from build123d import *

# Parameters (mm, degrees)
BOSS_EXTRU_1_DEPTH      = 6
ESQUISSE3_R             = 19
ENL_V_MAT_EXTRU_1_DEPTH = 10
ESQUISSE4_W             = 20
ESQUISSE4_H             = 60
ENL_V_MAT_EXTRU_2_DEPTH = 10
ESQUISSE5_W             = 20
ESQUISSE5_H             = 48
BOSS_EXTRU_2_DEPTH      = 6
ESQUISSE6_R             = 1.5
ENL_V_MAT_EXTRU_3_DEPTH = 10
ESQUISSE7_R             = 1.5
ENL_V_MAT_EXTRU_4_DEPTH = 10
ESQUISSE8_R             = 1.5
ENL_V_MAT_EXTRU_5_DEPTH = 10
ESQUISSE9_R             = 3.5
ESQUISSE9_R_2           = 1.5
ENL_V_MAT_EXTRU_6_DEPTH = 10
ESQUISSE10_R            = 1.5
ENL_V_MAT_EXTRU_7_DEPTH = 10
ESQUISSE11_R            = 1.5
ENL_V_MAT_EXTRU_8_DEPTH = 10
ESQUISSE13_R            = 5
ENL_V_MAT_EXTRU_9_DEPTH = 10


with BuildPart() as part:
    # Esquisse2 → Boss.-Extru.1 (new body)
    with BuildSketch(Plane.XY):
        Polygon((-82.846139514, -43.409107348), (-62.846139514, -43.409107348), (-62.846139514, -37.409107348), (-42.846139514, -37.409107348), (-42.846139514, -43.409107348), (-22.846139514, -43.409107348), (-22.846139514, -37.409107348), (-2.846139514, -37.409107348), (-2.846139514, -43.409107348), (17.153860486, -43.409107348), (17.153860486, -37.409107348), (37.153860486, -37.409107348), (37.153860486, -43.409107348), (57.153860486, -43.409107348), (57.153860486, -37.409107348), (77.153860486, -37.409107348), (77.153860486, -43.409107348), (97.153860486, -43.409107348), (97.153860486, -37.409107348), (117.153860486, -37.409107348), (117.153860486, -43.409107348), (137.153860486, -43.409107348), (137.153860486, -37.409107348), (157.153860486, -37.409107348), (157.153860486, -43.409107348), (177.153860486, -43.409107348), (177.153860486, -37.409107348), (197.153860486, -37.409107348), (197.153860486, -43.409107348), (217.153860486, -43.409107348), (217.153860486, -37.409107348), (237.153860486, -37.409107348), (237.153860486, -43.409107348), (257.153860486, -43.409107348), (257.153860486, -37.409107348), (277.153860486, -37.409107348), (277.153860486, -43.409107348), (297.153860486, -43.409107348), (297.153860486, -37.409107348), (317.153860486, -37.409107348), (317.153860486, -43.409107348), (337.153860486, -43.409107348), (337.153860486, 16.590892652), (317.153860486, 16.590892652), (317.153860486, 10.590892652), (297.153860486, 10.590892652), (297.153860486, 16.590892652), (277.153860486, 16.590892652), (277.153860486, 10.590892652), (257.153860486, 10.590892652), (257.153860486, 16.590892652), (237.153860486, 16.590892652), (237.153860486, 10.590892652), (217.153860486, 10.590892652), (217.153860486, 16.590892652), (197.153860486, 16.590892652), (197.153860486, 10.590892652), (177.153860486, 10.590892652), (177.153860486, 16.590892652), (157.153860486, 16.590892652), (157.153860486, 10.590892652), (137.153860486, 10.590892652), (137.153860486, 16.590892652), (117.153860486, 16.590892652), (117.153860486, 10.590892652), (97.153860486, 10.590892652), (97.153860486, 16.590892652), (77.153860486, 16.590892652), (77.153860486, 10.590892652), (57.153860486, 10.590892652), (57.153860486, 16.590892652), (37.153860486, 16.590892652), (37.153860486, 10.590892652), (17.153860486, 10.590892652), (17.153860486, 16.590892652), (-2.846139514, 16.590892652), (-2.846139514, 10.590892652), (-22.846139514, 10.590892652), (-22.846139514, 16.590892652), (-42.846139514, 16.590892652), (-42.846139514, 10.590892652), (-62.846139514, 10.590892652), (-62.846139514, 16.590892652), (-82.846139514, 16.590892652), align=None)
    extrude(amount=BOSS_EXTRU_1_DEPTH)

    # Esquisse3 → Enlèv. mat.-Extru.1 (cut)
    with BuildSketch(Plane.XY.offset(6)):
        with Locations((-37.846139514, -13.409107348)):
            Circle(ESQUISSE3_R)
    extrude(amount=-ENL_V_MAT_EXTRU_1_DEPTH, mode=Mode.SUBTRACT)

    # Esquisse4 → Enlèv. mat.-Extru.2 (cut)
    with BuildSketch(Plane.XY.offset(6)):
        with Locations((-72.846139514, -13.409107348)):
            Rectangle(ESQUISSE4_W, ESQUISSE4_H)
    extrude(amount=-ENL_V_MAT_EXTRU_2_DEPTH, mode=Mode.SUBTRACT)

    # Esquisse5 → Boss.-Extru.2 (add)
    with BuildSketch(Plane.XY.offset(6)):
        with Locations((347.153860486, -13.409107348)):
            Rectangle(ESQUISSE5_W, ESQUISSE5_H)
    extrude(amount=-BOSS_EXTRU_2_DEPTH)

    # Esquisse6 → Enlèv. mat.-Extru.3 (cut)
    with BuildSketch(Plane.XY.offset(6)):
        with Locations((127.153860486, -40.409107348)):
            Circle(ESQUISSE6_R)
        with Locations((287.153860486, -40.409107348)):
            Circle(ESQUISSE6_R)
        with Locations((7.153860486, -40.409107348)):
            Circle(ESQUISSE6_R)
        with Locations((7.153860486, 13.590892652)):
            Circle(ESQUISSE6_R)
        with Locations((127.153860486, 13.590892652)):
            Circle(ESQUISSE6_R)
        with Locations((287.153860486, 13.590892652)):
            Circle(ESQUISSE6_R)
    extrude(amount=-ENL_V_MAT_EXTRU_3_DEPTH, mode=Mode.SUBTRACT)

    # Esquisse7 → Enlèv. mat.-Extru.4 (cut)
    with BuildSketch(Plane.XY.offset(6)):
        with Locations((-59.846139514, -13.409107348)):
            Circle(ESQUISSE7_R)
    extrude(amount=-ENL_V_MAT_EXTRU_4_DEPTH, mode=Mode.SUBTRACT)

    # Esquisse8 → Enlèv. mat.-Extru.5 (cut)
    with BuildSketch(Plane.XY.offset(6)):
        with Locations((354.153860486, -13.409107348)):
            Circle(ESQUISSE8_R)
    extrude(amount=-ENL_V_MAT_EXTRU_5_DEPTH, mode=Mode.SUBTRACT)

    # Esquisse9 → Enlèv. mat.-Extru.6 (cut)
    with BuildSketch(Plane.XY.offset(6)):
        with Locations((1.153860486, -13.409107348)):
            Circle(ESQUISSE9_R)
        with Locations((-7.096139514, -13.409107348)):
            Circle(ESQUISSE9_R_2)
        with Locations((9.403860486, -13.409107348)):
            Circle(ESQUISSE9_R_2)
    extrude(amount=-ENL_V_MAT_EXTRU_6_DEPTH, mode=Mode.SUBTRACT)

    # Esquisse10 → Enlèv. mat.-Extru.7 (cut)
    with BuildSketch(Plane.XY.offset(6)):
        with Locations((-32.846139514, 13.590892652)):
            Circle(ESQUISSE10_R)
        with Locations((-32.846139514, -40.409107348)):
            Circle(ESQUISSE10_R)
    extrude(amount=-ENL_V_MAT_EXTRU_7_DEPTH, mode=Mode.SUBTRACT)

    # Esquisse11 → Enlèv. mat.-Extru.8 (cut)
    with BuildSketch(Plane.XY.offset(6)):
        with Locations((87.153860486, 13.590892652)):
            Circle(ESQUISSE11_R)
        with Locations((87.153860486, -40.409107348)):
            Circle(ESQUISSE11_R)
    extrude(amount=-ENL_V_MAT_EXTRU_8_DEPTH, mode=Mode.SUBTRACT)

    # Esquisse13 → Enlèv. mat.-Extru.9 (cut)
    with BuildSketch(Plane.XY.offset(6)):
        with Locations((332.153860486, -13.409107348)):
            Circle(ESQUISSE13_R)
    extrude(amount=-ENL_V_MAT_EXTRU_9_DEPTH, mode=Mode.SUBTRACT)


solid = part.part
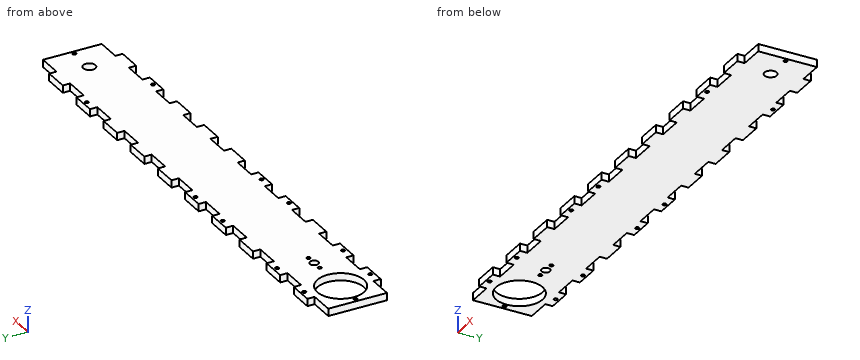
Can you work these out from the model? Positions are in its coordinate system, mm. Round coordinates to 2 decimals unless told otherwise and drop trailing zeros. Order: outer loops, then holes, each group sorted by start corner. A loop starts at its lowest first (then second) coordinate and runs counter-clockwise, first axis right, second up. Notation, with made-up numbers: (21, 12.25) -> (29, 12.25) arc R17 cw to (29, 32.25) -> close; hole circle Ø5 at (48, -34.5). An arc over 180 degrees is marked (long way). Write each question's results on one line, items separated by ' | '. Start each with the question number.
Item 1: If we section it at C-C, the plane z = 3.5: State how many separate pieces and enclosed holes the cut face has, then the cut area to 3 significant figures.
Item 2: Please list where these lines run through material, in increasing order: L1, parallel to Y at x = 77, z = 1.75; L2, parallel to X at y = -16, z = 2.3; L3, parallel to X at y = 2, z = 0.5.
Item 3: If we section it at B-B, the plane x = 25.5: Write out the boundary of the cut face in (y, z), then the cut area to 3 significant figures.
Item 4: If we section it at A-A, the plane y = -22.5: Write out the boundary of the cut face in (x, z).
Item 5: Will these pins go through, and if not, where does the flat tip stop? pin 1 (3 mm diameter, centred on y = 14.5, z = 3, fed in from -X); pin 2 (3 mm diameter, centred on x = 224.5, z = 3.5, fed in from -Y); pin 3 (3 mm diameter, centred on x = 146, z = 4, fed in from +Y).
Results:
1) separate pieces: 1 | enclosed holes: 17 | area: 21,200 mm2
2) L1: y = -37.41 to 10.59 | L2: x = -62.85 to -56.67, -19.02 to -1.2, 3.51 to 327.88, 336.43 to 357.15 | L3: x = -62.85 to -48.96, -26.73 to 357.15
3) outline: (-37.41, 0) -> (10.59, 0) -> (10.59, 6) -> (-37.41, 6) -> close | area: 288 mm2
4) outline: (-62.85, 0) -> (-54.53, 0) -> (-54.53, 6) -> (-62.85, 6) -> close; (-21.16, 0) -> (357.15, 0) -> (357.15, 6) -> (-21.16, 6) -> close
5) pin 1: stops at x = -42.85 | pin 2: stops at y = -37.41 | pin 3: stops at y = 10.59
